Build history of the part. All positions in model axes, mm. Face numbers are marked on the shaded views. A direction names the side the tool comes from. Give positions to 0.01 mm unless a question says otherwise; leave off trailing zeros. Write each loop counter-clockwise with the first axis right and the second up, starting at its lowest first coordinate (ties: lowest second). Pieces come first, ordered by that corner, then holes. Notation, with made-up numbers: (71.5, 76.5) -> (111.5, 76.5) arc R22 ccw to (111.5, 94.5) -> close; hole circle Ø1 at (42.25, 15.25). An arc over 180 degrees is marked (long way). Put each result on its own line as item: value.
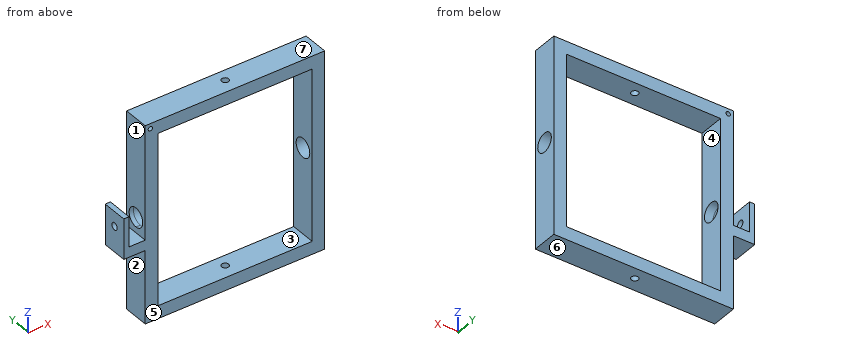
from build123d import *

# Parameters (mm, degrees)
SKETCH1_W            = 230
SKETCH1_H            = 230
SKETCH1_W_2          = 200
SKETCH1_H_2          = 200
BOSS_EXTRUDE1_DEPTH  = 30
SKETCH2_R            = 11
CUT_EXTRUDE3_DEPTH   = 206
SKETCH3_W            = 12.648408852
SKETCH3_H            = 30
BOSS_EXTRUDE2_DEPTH  = 28
SKETCH4_W            = 33.277006623
SKETCH4_H            = 30
BOSS_EXTRUDE4_DEPTH  = 41
SKETCH6_R            = 4
CUT_EXTRUDE4_DEPTH   = 218
SKETCH8_R            = 4.046690546
CUT_EXTRUDE6_DEPTH   = 280
CUT_EXTRUDE7_START   = -230
SKETCH9_R            = 11
CUT_EXTRUDE7_DEPTH   = 230
SKETCH11_W           = 19.776160892
SKETCH11_H           = 30
CUT_EXTRUDE8_DEPTH   = 41
SKETCH12_R           = 4
CUT_EXTRUDE9_DEPTH   = 264
SKETCH13_R           = 4
CUT_EXTRUDE10_DEPTH  = 264
SKETCH15_W           = 8.223839108
SKETCH15_H           = 30
CUT_EXTRUDE11_DEPTH  = 64
SKETCH16_W           = 6.512440182
SKETCH16_H           = 30
BOSS_EXTRUDE5_DEPTH  = 40
SKETCH17_R           = 4
CUT_EXTRUDE12_DEPTH  = 276
SKETCH18_W           = 10.028465144
SKETCH18_H           = 30
BOSS_EXTRUDE6_DEPTH  = 203
SKETCH19_W           = 9.920001469
SKETCH19_H           = 30
BOSS_EXTRUDE7_DEPTH  = 203
SKETCH21_W           = 19.776160892
SKETCH21_H           = 30
CUT_EXTRUDE13_DEPTH  = 203
SKETCH22_W           = 10.441032334
SKETCH22_H           = 30
CUT_EXTRUDE14_DEPTH  = 278
SKETCH23_W           = 4.062093177
SKETCH23_H           = 12.100968139
BOSS_EXTRUDE8_DEPTH  = 30
SKETCH24_W           = 9.989580678
SKETCH24_H           = 30
CUT_EXTRUDE15_DEPTH  = 248
CUT_EXTRUDE16_START  = -248
SKETCH25_R           = 11
CUT_EXTRUDE16_DEPTH  = 248
SKETCH26_W           = 12.005407817
SKETCH26_H           = 30
BOSS_EXTRUDE9_DEPTH  = 25
SKETCH27_W           = 9.568763957
SKETCH27_H           = 30
BOSS_EXTRUDE10_DEPTH = 35
SKETCH28_W           = 3.507869301
SKETCH28_H           = 30
CUT_EXTRUDE17_DEPTH  = 35
SKETCH29_R           = 4.25
CUT_EXTRUDE18_DEPTH  = 257
SKETCH33_R           = 2.5
CUT_EXTRUDE20_DEPTH  = 44


with BuildPart() as part:
    # Sketch1 → Boss-Extrude1 (new body)
    with BuildSketch(Plane(origin=(0, 0, 0), x_dir=(1, 0, 0), z_dir=(0, 1, 0))):
        Rectangle(SKETCH1_W, SKETCH1_H)
        Rectangle(SKETCH1_W_2, SKETCH1_H_2, mode=Mode.SUBTRACT)
    extrude(amount=BOSS_EXTRUDE1_DEPTH)

    # Sketch2 → Cut-Extrude3 (cut)
    with BuildSketch(Plane(origin=(115, 0, 0), x_dir=(0, 0, -1), z_dir=(1, 0, 0))):
        with Locations((0, 15)):
            Circle(SKETCH2_R)
    extrude(amount=-CUT_EXTRUDE3_DEPTH, mode=Mode.SUBTRACT)

    # Sketch3 → Boss-Extrude2 (add)
    with BuildSketch(Plane(origin=(115, 0, 0), x_dir=(0, 0, -1), z_dir=(1, 0, 0))):
        with Locations((26.610788675, 15)):
            Rectangle(SKETCH3_W, SKETCH3_H)
    extrude(amount=BOSS_EXTRUDE2_DEPTH)

    # Sketch4 → Boss-Extrude4 (add)
    with BuildSketch(Plane.XY.offset(-20.286584249)):
        with Locations((126.361496689, 15)):
            Rectangle(SKETCH4_W, SKETCH4_H)
    extrude(amount=BOSS_EXTRUDE4_DEPTH)

    # Sketch6 → Cut-Extrude4 (cut)
    with BuildSketch(Plane.ZY.offset(115)):
        with Locations((0, 15)):
            Circle(SKETCH6_R)
    extrude(amount=-CUT_EXTRUDE4_DEPTH, mode=Mode.SUBTRACT)

    # Sketch8 → Cut-Extrude6 (cut)
    with BuildSketch(Plane.XY.offset(115)):
        with Locations((0, 16.175919114)):
            Circle(SKETCH8_R)
    extrude(amount=-CUT_EXTRUDE6_DEPTH, mode=Mode.SUBTRACT)

    # Sketch9 → Cut-Extrude7 (cut)
    with BuildSketch(Plane.ZY.offset(115).offset(CUT_EXTRUDE7_START)):
        with Locations((0, 15)):
            Circle(SKETCH9_R)
    extrude(amount=CUT_EXTRUDE7_DEPTH, mode=Mode.SUBTRACT)

    # Sketch11 → Cut-Extrude8 (cut)
    with BuildSketch(Plane.XY.offset(20.713415751)):
        with Locations((124.888080446, 15)):
            Rectangle(SKETCH11_W, SKETCH11_H)
    extrude(amount=-CUT_EXTRUDE8_DEPTH, mode=Mode.SUBTRACT)

    # Sketch12 → Cut-Extrude9 (cut)
    with BuildSketch(Plane.ZY.offset(115)):
        with Locations((0, 15)):
            Circle(SKETCH12_R)
    extrude(amount=-CUT_EXTRUDE9_DEPTH, mode=Mode.SUBTRACT)

    # Sketch13 → Cut-Extrude10 (cut)
    with BuildSketch(Plane(origin=(0, 30, 0), x_dir=(1, 0, 0), z_dir=(0, 1, 0))):
        with Locations(Location((106.851068212, -106.17718303, 0), (0, 0, 270))):
            Circle(SKETCH13_R)
    extrude(amount=-CUT_EXTRUDE10_DEPTH, mode=Mode.SUBTRACT)

    # Sketch15 → Cut-Extrude11 (cut)
    with BuildSketch(Plane.XY.offset(20.713415751)):
        with Locations((138.888080446, 15)):
            Rectangle(SKETCH15_W, SKETCH15_H)
    extrude(amount=-CUT_EXTRUDE11_DEPTH, mode=Mode.SUBTRACT)

    # Sketch16 → Boss-Extrude5 (add)
    with BuildSketch(Plane.XY.offset(-20.286584249)):
        with Locations((131.519940801, 15)):
            Rectangle(SKETCH16_W, SKETCH16_H)
    extrude(amount=BOSS_EXTRUDE5_DEPTH)

    # Sketch17 → Cut-Extrude12 (cut)
    with BuildSketch(Plane.ZY.offset(115)):
        with Locations((0, 15)):
            Circle(SKETCH17_R)
    extrude(amount=-CUT_EXTRUDE12_DEPTH, mode=Mode.SUBTRACT)

    # Sketch18 → Boss-Extrude6 (add)
    with BuildSketch(Plane(origin=(0, 0, 100), x_dir=(-1, 0, 0), z_dir=(0, 0, -1))):
        with Locations((-94.985767428, 15)):
            Rectangle(SKETCH18_W, SKETCH18_H)
    extrude(amount=BOSS_EXTRUDE6_DEPTH)

    # Sketch19 → Boss-Extrude7 (add)
    with BuildSketch(Plane(origin=(0, 0, 100), x_dir=(-1, 0, 0), z_dir=(0, 0, -1))):
        with Locations((95.039999266, 15)):
            Rectangle(SKETCH19_W, SKETCH19_H)
    extrude(amount=BOSS_EXTRUDE7_DEPTH)

    # Sketch21 → Cut-Extrude13 (cut)
    with BuildSketch(Plane(origin=(0, 0, -32.934993101), x_dir=(-1, 0, 0), z_dir=(0, 0, -1))):
        with Locations((-124.888080446, 15)):
            Rectangle(SKETCH21_W, SKETCH21_H)
    extrude(amount=-CUT_EXTRUDE13_DEPTH, mode=Mode.SUBTRACT)

    # Sketch22 → Cut-Extrude14 (cut)
    with BuildSketch(Plane(origin=(0, 0, -115), x_dir=(-1, 0, 0), z_dir=(0, 0, -1))):
        with Locations((-109.779483833, 15)):
            Rectangle(SKETCH22_W, SKETCH22_H)
    extrude(amount=-CUT_EXTRUDE14_DEPTH, mode=Mode.SUBTRACT)

    # Sketch23 → Boss-Extrude8 (add)
    with BuildSketch(Plane(origin=(0, 30, 0), x_dir=(1, 0, 0), z_dir=(0, 1, 0))):
        with Locations((102.527921077, -108.949515931)):
            Rectangle(SKETCH23_W, SKETCH23_H)
    extrude(amount=-BOSS_EXTRUDE8_DEPTH)

    # Sketch24 → Cut-Extrude15 (cut)
    with BuildSketch(Plane(origin=(0, 0, -115), x_dir=(-1, 0, 0), z_dir=(0, 0, -1))):
        with Locations((110.005209661, 15)):
            Rectangle(SKETCH24_W, SKETCH24_H)
    extrude(amount=-CUT_EXTRUDE15_DEPTH, mode=Mode.SUBTRACT)

    # Sketch25 → Cut-Extrude16 (cut)
    with BuildSketch(Plane.ZY.offset(105.010419322).offset(CUT_EXTRUDE16_START)):
        with Locations(Location((0, 15, 0), (0, 0, 180))):
            Circle(SKETCH25_R)
    extrude(amount=CUT_EXTRUDE16_DEPTH, mode=Mode.SUBTRACT)

    # Sketch26 → Boss-Extrude9 (add)
    with BuildSketch(Plane.ZY.offset(105.010419322)):
        with Locations((-23.736715717, 15)):
            Rectangle(SKETCH26_W, SKETCH26_H)
    extrude(amount=BOSS_EXTRUDE9_DEPTH)

    # Sketch27 → Boss-Extrude10 (add)
    with BuildSketch(Plane.XY.offset(-17.734011808)):
        with Locations((-125.226037344, 15)):
            Rectangle(SKETCH27_W, SKETCH27_H)
    extrude(amount=BOSS_EXTRUDE10_DEPTH)

    # Sketch28 → Cut-Extrude17 (cut)
    with BuildSketch(Plane.XY.offset(17.265988192)):
        with Locations((-122.195590016, 15)):
            Rectangle(SKETCH28_W, SKETCH28_H)
    extrude(amount=-CUT_EXTRUDE17_DEPTH, mode=Mode.SUBTRACT)

    # Sketch29 → Cut-Extrude18 (cut)
    with BuildSketch(Plane(origin=(104.558967666, 0, 0), x_dir=(0, 0, -1), z_dir=(1, 0, 0))):
        with Locations((0, 15)):
            Circle(SKETCH29_R)
    extrude(amount=-CUT_EXTRUDE18_DEPTH, mode=Mode.SUBTRACT)

    # Sketch33 → Cut-Extrude20 (cut)
    with BuildSketch(Plane(origin=(0, 0, 0), x_dir=(-1, 0, 0), z_dir=(0, -1, 0))):
        with Locations(Location((99.023642446, -109.086175653, 0), (0, 0, 90))):
            Circle(SKETCH33_R)
    extrude(amount=-CUT_EXTRUDE20_DEPTH, mode=Mode.SUBTRACT)


solid = part.part
1) Wall check: L1, parallel to X at y = 18.25, z = -17; L2, parallel to X at y = 21, z = -98; L3, parallel to Y at x = 95, z = 0. Give the ranges that are in metal, low to high.
Filled sheet:
L1: -130.01 to -123.95, -105.01 to -90.08, 89.97 to 104.56
L2: -105.01 to -90.08, 89.97 to 104.56
L3: 0 to 4, 26 to 30
2) Slice it at C-C (x = -48). Write the cut outline in (y, z), plus the area to 3 significant figures.
Filled sheet:
outline: (0, -115) -> (30, -115) -> (30, -100) -> (0, -100) -> close; (0, 100) -> (30, 100) -> (30, 115) -> (0, 115) -> close
area: 900 mm2
3) Slice it at B-B (x = 0). Write the cut outline in (y, z).
Filled sheet:
outline: (0, -115) -> (12.13, -115) -> (12.13, -100) -> (0, -100) -> close; (0, 100) -> (12.13, 100) -> (12.13, 115) -> (0, 115) -> close; (20.22, -115) -> (30, -115) -> (30, -100) -> (20.22, -100) -> close; (20.22, 100) -> (30, 100) -> (30, 115) -> (20.22, 115) -> close
4) Pin check, flat tips, straight feed: pin 1 (15 mm diameter, centred on y = 22.5, z = 21.5, fed in from -X); pin 2 (5 mm diameter, centred on x = -128.5, y = 20, fed in from +Z); pin 3 (4 mm diameter, centred on y = 7, z = 38.5, fed in from -X). Stop position of each tip, or through.
Filled sheet:
pin 1: x = -130.01
pin 2: z = 17.27
pin 3: x = -105.01
5) Tool access for the marked faces 1, 2 and 3: list every direction of +Z, -Z, +X, -X, +Y, -Y with a clear straight run to the whole face (end or side of a thin tool).
Filled sheet:
face 1: +Z, +Y, -Y
face 2: -Z, -X, +Y, -Y
face 3: +Y, -Y
6) Slice it at D-D (z = -36.5). Write the cut outline in (x, y), plus the area to 3 significant figures.
Filled sheet:
outline: (-105.01, 0) -> (-90.08, 0) -> (-90.08, 30) -> (-105.01, 30) -> close; (89.97, 0) -> (104.56, 0) -> (104.56, 30) -> (89.97, 30) -> close
area: 886 mm2
7) Pull direction Z, two halves, no side cores. Call the marked faces 4, 5, 6 and 7: released by +Z, released by -Z, zero draft, split by the parting line, or undercut.
Filled sheet:
face 4: undercut
face 5: zero draft
face 6: released by -Z
face 7: released by +Z
8) Slice it at A-A (z = 0). Write the cut outline in (x, y).
Filled sheet:
outline: (-130.01, 0) -> (-123.95, 0) -> (-123.95, 10.75) -> (-130.01, 10.75) -> close; (-130.01, 19.25) -> (-123.95, 19.25) -> (-123.95, 30) -> (-130.01, 30) -> close; (-105.01, 0) -> (-90.08, 0) -> (-90.08, 4) -> (-105.01, 4) -> close; (-105.01, 26) -> (-90.08, 26) -> (-90.08, 30) -> (-105.01, 30) -> close; (89.97, 0) -> (104.56, 0) -> (104.56, 4) -> (89.97, 4) -> close; (89.97, 26) -> (104.56, 26) -> (104.56, 30) -> (89.97, 30) -> close
